Design review of the part shown in the three views and the two pictorial views. Dimensions are in mm from the part's minimum x, y and z. Give positions to 0.01 mm unless a question says otherwise; leave off trailing zeros. Loops run counter-clockwise (first coordinate to the right, second up) from the corner with the lowest first, then second, coordinate; pieces in that order, holes last. Notation, with made-up numbers: (-18, -21.5) - (6, -21.5) arc R7 cw to (6, -12.5) - close; hole circle Ø3 at (32.5, -5). An arc over 180 degrees is marked (long way). Answer in a Markdown table with one row per item.
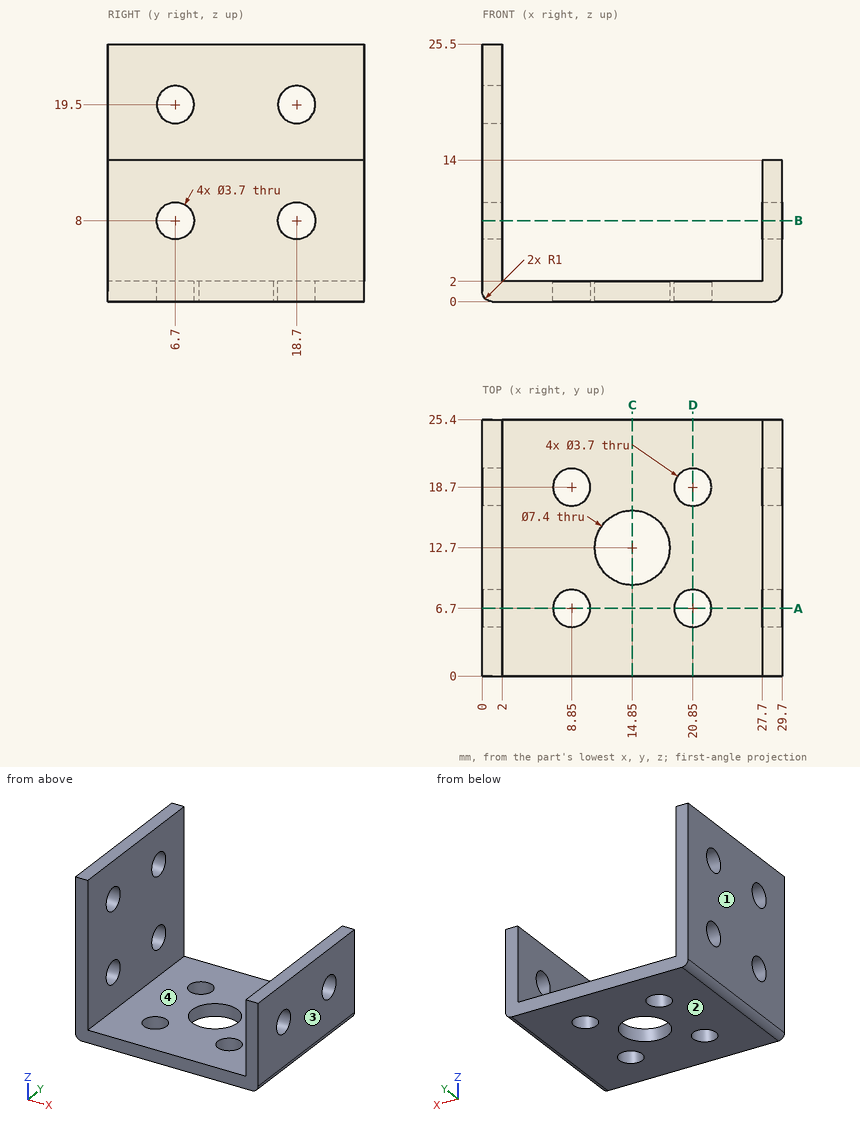
1. We need section B-B, the plane z = 8. Give the boundary of the cut face in (x, y).
Values:
| item | result |
|---|---|
| outline | (0, 0) - (2, 0) - (2, 4.85) - (0, 4.85) - close; (0, 8.55) - (2, 8.55) - (2, 16.85) - (0, 16.85) - close; (0, 20.55) - (2, 20.55) - (2, 25.4) - (0, 25.4) - close; (27.7, 0) - (29.7, 0) - (29.7, 4.85) - (27.7, 4.85) - close; (27.7, 8.55) - (29.7, 8.55) - (29.7, 16.85) - (27.7, 16.85) - close; (27.7, 20.55) - (29.7, 20.55) - (29.7, 25.4) - (27.7, 25.4) - close |
2. Clearance check with flat-ended pins moving along their axes: pin 1 (3 mm diameter, centred on x = 17.5, y = 2.5, fed in from +Z); pin 2 (1.6 mm diameter, centred on x = 29, y = 15.5, fed in from +Z). State where each tip first meets the part, or that it passes through.
Values:
| item | result |
|---|---|
| pin 1 | stops at z = 2 |
| pin 2 | stops at z = 14 |
3. We need section A-A, the plane y = 6.7. Count the separate pieces of the cut face and the enclosed holes in it, and give its area (3 significant figures).
Values:
| item | result |
|---|---|
| separate pieces | 6 |
| enclosed holes | 0 |
| area | 93.0 mm^2 |
4. Wall thickness on line 1 (Y direction, x = 20.85, z = 0.75); line 2 (X direction, y = 24, z = 12.5); line 3 (X direction, y = 18.25, z = 1.25): over which ranges is each line inside the solid? List them lowest first. Write a range as [from, to].
Values:
| item | result |
|---|---|
| line 1 | y = [0, 4.85], [8.55, 16.85], [20.55, 25.4] |
| line 2 | x = [0, 2], [27.7, 29.7] |
| line 3 | x = [0, 7.06], [10.64, 19.06], [22.64, 29.7] |
5. We need section C-C, the plane x = 14.85. Give the boundary of the cut face in (y, z), and give its area (3 significant figures).
Values:
| item | result |
|---|---|
| outline | (0, 0) - (9, 0) - (9, 2) - (0, 2) - close; (16.4, 0) - (25.4, 0) - (25.4, 2) - (16.4, 2) - close |
| area | 36.0 mm^2 |
6. Mouldability with a two-part tool opening along X and no side actions: class the marked faces 1, 2, 3 and 4 as released by +X, released by -X, zero draft, split by the parting line, or undercut.
Values:
| item | result |
|---|---|
| face 1 | released by -X |
| face 2 | zero draft |
| face 3 | released by +X |
| face 4 | undercut |
7. We need section D-D, the plane x = 20.85. Give the boundary of the cut face in (y, z).
Values:
| item | result |
|---|---|
| outline | (0, 0) - (4.85, 0) - (4.85, 2) - (0, 2) - close; (8.55, 0) - (16.85, 0) - (16.85, 2) - (8.55, 2) - close; (20.55, 0) - (25.4, 0) - (25.4, 2) - (20.55, 2) - close |
